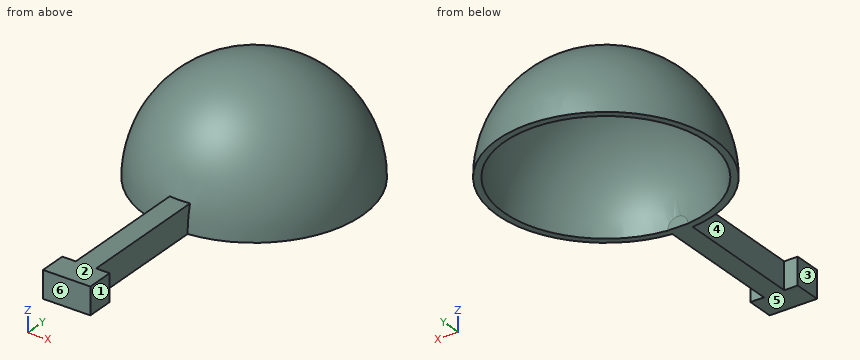
from build123d import *

# Parameters (mm, degrees)
REVOLUTION_ANGLE = 180
PAD_DEPTH        = 4


with BuildPart() as part:
    # Sketch → Revolution (revolve)
    with BuildSketch(Plane.XY):
        with BuildLine():
            ThreePointArc((16, 0), (0, 16), (-16, 0))
            Line((-16, 0), (-15, 0))
            ThreePointArc((15, 0), (0, 15), (-15, 0))
            Line((15, 0), (16, 0))
        make_face()
    revolve(axis=Axis((0, 0, 0), (1, 0, 0)), revolution_arc=REVOLUTION_ANGLE)

    # Sketch001 → Pad (new body)
    with BuildSketch(Plane(origin=(0, 0, 0), x_dir=(1, 0, 0), z_dir=(0, 0, -1))):
        Polygon((-1.5, 14.924812), (-1.5, 34.924812), (-3.5, 34.924812), (-3.5, 38.924812), (3.5, 38.924812), (3.5, 34.924812), (1.5, 34.924812), (1.5, 14.924812), align=None)
    extrude(amount=-PAD_DEPTH)


solid = part.part
Design review of the part built by this model. Coordinates are the model's own, in mm. Face numbers are marked on the shaded views. A direction names the side the tool comes from. Give positions to 0.01 mm unless a question says otherwise; leave off trailing zeros. Order: outer loops, then holes, each group sorted by start corner. A loop starts at its lowest first (then second) coordinate and runs counter-clockwise, first axis right, second up.
1. To check wall thickness, follow L1, parallel to Y at x = 9, z = 7.5; L2, parallel to Y at x = -8, z = 7; L3, parallel to Z at x = 1.5, y = -35.5. State the ranges of each line that lie inside material, in increasing order.
Solution:
L1: y = -10.9 to -9.37, 9.37 to 10.9
L2: y = -11.96 to -10.58, 10.58 to 11.96
L3: z = 0 to 4
2. Add section B-B, the plane z = 8.5. State the section outline as (x, y) points.
Solution:
outline: circle Ø27.11 at (0, 0); hole circle Ø24.72 at (0, 0)
3. Add section A-A, the plane y = -24. State the section outline as (x, z) points, then the cut area to 3 significant figures.
Solution:
outline: (-1.5, 0) - (1.5, 0) - (1.5, 4) - (-1.5, 4) - close
area: 12.0 mm2
4. For pin 1 Ø0.7 at (x, z) = (0, 0.5) entering from +Y; pin 2 Ø7.5 at (x, y) = (0, -27) entering from +Z; pin 3 Ø4.5 at (y, z) = (-23.5, 3) entering from -X, all flat-tipped, find the tip position at first contact; note any pin that passes through.
Solution:
pin 1: stops at y = 16
pin 2: stops at z = 4
pin 3: stops at x = -1.5
5. Mouldability with a two-part tool opening along Y and no side actions: class the marked faces 4, 5 and 6 as +Y half, -Y half, draft (parallel to the pull), parting line (faces both ways), or undercut.
Solution:
face 4: undercut
face 5: draft
face 6: -Y half
6. Add section C-C, the plane x = -12.5. State the section outline as (y, z) points.
Solution:
outline: (-9.99, 0) - (-8.29, 0) arc R8.29 cw to (8.29, 0) - (9.99, 0) arc R9.99 ccw to start
7. Tool access review of the marked faces 1, 2 and 3: name each direction out of +Z, -Z, +X, -X, +Y, -Y from which nothing blocks a thin tool from reaching the whole face with its end or side.
Solution:
face 1: +Z, -Z, +X, -Y
face 2: +Z, +X, -X, -Y
face 3: +Z, -Z, -X, -Y
